Geometry check sheet. Reference: the model listing, model coordinates, mm. A direction names the side the tool comes from. Coordinates: 2 decimals unless noted, no trailing zeros. Loops run counter-clockwise (first coordinate to the right, second up) from the corner with the lowest first, then second, coordinate; pieces in that order, holes last.
from build123d import *

# Parameters (mm, degrees)
F0_R     = 1.7272
F0_R_2   = 3.96875
F0_R_3   = 11.1125
F1_DEPTH = 3.175
F3_DEPTH = 3.175
F4_COUNT = 6
F4_ANGLE = 300


with BuildPart() as f1:
    # F0 (on Top) → F1 (new body)
    with BuildSketch(Plane.XY):
        with BuildLine():
            Line((-303.6125627, 32.54375), (-346.1094200534, 21.5120031198))
            ThreePointArc((-346.1094200534, 21.5120031198), (-362.7501254, 0), (-346.1094200534, -21.5120031198))
            Line((-346.1094200534, -21.5120031198), (-303.6125627, -32.54375))
            Line((-303.6125627, -32.54375), (-297.2625627, -32.54375))
            Line((-297.2625627, -32.54375), (-297.2625627, -29.36875))
            Line((-297.2625627, -29.36875), (-43.2625627, -29.36875))
            Line((-43.2625627, -29.36875), (-43.2625627, -32.54375))
            Line((-43.2625627, -32.54375), (-36.9125627, -32.54375))
            Line((-36.9125627, -32.54375), (-9.2338657221, -25.3586450757))
            ThreePointArc((-9.2338657221, -25.3586450757), (26.9875, 0), (-9.2338657221, 25.3586450757))
            Line((-9.2338657221, 25.3586450757), (-36.9125627, 32.54375))
            Line((-36.9125627, 32.54375), (-43.2625627, 32.54375))
            Line((-43.2625627, 32.54375), (-43.2625627, 29.36875))
            Line((-43.2625627, 29.36875), (-297.2625627, 29.36875))
            Line((-297.2625627, 29.36875), (-297.2625627, 32.54375))
            Line((-297.2625627, 32.54375), (-303.6125627, 32.54375))
        make_face()
        with Locations((-282.9750627, -24.60625)):
            Circle(F0_R, mode=Mode.SUBTRACT)
        with Locations((-352.3117115589, -11.7865861589)):
            Circle(F0_R, mode=Mode.SUBTRACT)
        with Locations((-328.7385392411, -11.7865861589)):
            Circle(F0_R_2, mode=Mode.SUBTRACT)
        with Locations((-57.5500627, -24.60625)):
            Circle(F0_R, mode=Mode.SUBTRACT)
        with Locations((-11.7865861589, -11.7865861589)):
            Circle(F0_R_2, mode=Mode.SUBTRACT)
        with Locations((11.7865861589, -11.7865861589)):
            Circle(F0_R, mode=Mode.SUBTRACT)
        with Locations((-340.5251254, 0)):
            Circle(F0_R_3, mode=Mode.SUBTRACT)
        with Locations((-289.7251254, 0)):
            Circle(F0_R, mode=Mode.SUBTRACT)
        with Locations((-352.3117115589, 11.7865861589)):
            Circle(F0_R_2, mode=Mode.SUBTRACT)
        with Locations((-328.7385392411, 11.7865861589)):
            Circle(F0_R, mode=Mode.SUBTRACT)
        with Locations((-282.9750627, 24.60625)):
            Circle(F0_R, mode=Mode.SUBTRACT)
        with Locations((-50.8, 0)):
            Circle(F0_R, mode=Mode.SUBTRACT)
        Circle(F0_R_3, mode=Mode.SUBTRACT)
        with Locations((-11.7865861589, 11.7865861589)):
            Circle(F0_R, mode=Mode.SUBTRACT)
        with Locations((11.7865861589, 11.7865861589)):
            Circle(F0_R_2, mode=Mode.SUBTRACT)
        with Locations((-57.5500627, 24.60625)):
            Circle(F0_R, mode=Mode.SUBTRACT)
    extrude(amount=F1_DEPTH)

    # F2 (on face) → F3 (cut, through all)
    with BuildSketch(Plane(origin=(0, 0, 0), x_dir=(1, 0, 0), z_dir=(0, 0, -1))):
        with BuildLine():
            ThreePointArc((-348.3828495059, -7.8577241059), (-350.1488326996, -5.55625), (-351.2589761446, -2.8761266387))
            Line((-351.2589761446, -2.8761266387), (-352.0256797693, -3.0815642558))
            ThreePointArc((-352.0256797693, -3.0815642558), (-350.8362403638, -5.953125), (-348.9441155135, -8.4189901135))
            Line((-348.9441155135, -8.4189901135), (-348.3828495059, -7.8577241059))
        make_face()
    f3 = extrude(amount=-F3_DEPTH, mode=Mode.SUBTRACT)

    # F4: F3 ×6 about axis
    f4_axis = Axis((-340.5251254, 0, 0), (0, 0, -1))
    for i in range(1, F4_COUNT):
        add(f3.rotate(f4_axis, i * F4_ANGLE / (F4_COUNT - 1)), mode=Mode.SUBTRACT)


solid = f1.part
(1) Sectioned sample at B-B on z = 0.9. State how many separate pieces and enclosed holes the cut face has, and give its area (3 significant figures).
Findings:
separate pieces: 1
enclosed holes: 16
area: 20,700 mm2
(2) Access from +Z, -Z, +X, -X, +Y, -Y to the whole of each face (thin tool, end or side, straight path). Record for faces 5 (the cylindrical face through (-362.746, 0.41, 1.565)), 6 (the flat face through (-22.88, 28.9, 1.57)).
Findings:
face 5: +Z, -Z, -X
face 6: +Z, -Z, +Y
(3) Scan lines: L1, parallel to X at y = -0.5, z = 0.7; L2, parallel to Y at x = -155, z = 1.8; L3, parallel to X at y = -9.5, z = 0.65. Record each from-to range of solid material in increasing order.
Findings:
L1: x = -362.74 to -351.63, -329.42 to -291.38, -288.07 to -52.45, -49.15 to -11.1, 11.1 to 26.98
L2: y = -29.37 to 29.37
L3: x = -360.62 to -346.29, -334.76 to -331.98, -325.49 to -15.03, -8.54 to -5.77, 5.77 to 25.26
(4) Gauge pin test, flat ends, axial feed: pin 1 Ø1.5 at (y, z) = (10.5, 1) entering from +X; pin 2 Ø1.5 at (y, z) = (-20, 2.5) entering from -X; pin 3 Ø1.6 at (x, z) = (-129.5, 2) entering from -Y. Record the tip position at first contact, or that the pin passes through.
Findings:
pin 1: stops at x = 25.16
pin 2: stops at x = -351.63
pin 3: stops at y = -29.37
(5) Draft check along Y on faces 1 (the flat face through (-23.267, -29.001, 1.565)), 2 (the flat face through (-171, 0, 3.175)), 3 (the cylindrical face through (-356.277, 11.961, 1.565)), 4 (the cylindrical face through (26.978, -0.725, 1.565)). Enter one of: +Y half, -Y half, draft (parallel to the pull), parting line (faces both ways), or undercut.
Findings:
face 1: -Y half
face 2: draft
face 3: undercut
face 4: parting line
(6) Sectioned sample at A-A on x = 0. Record the cut outline in (y, z) (1 decimal), and give its area (3 significant figures).
Findings:
outline: (-27, 0) - (-11.1, 0) - (-11.1, 3.2) - (-27, 3.2) - close; (11.1, 0) - (27, 0) - (27, 3.2) - (11.1, 3.2) - close
area: 101 mm2
(7) Sectioned sample at C-C on x = -258. Record the cut outline in (y, z) (3 decimals).
Findings:
outline: (-29.369, 0) - (29.369, 0) - (29.369, 3.175) - (-29.369, 3.175) - close
